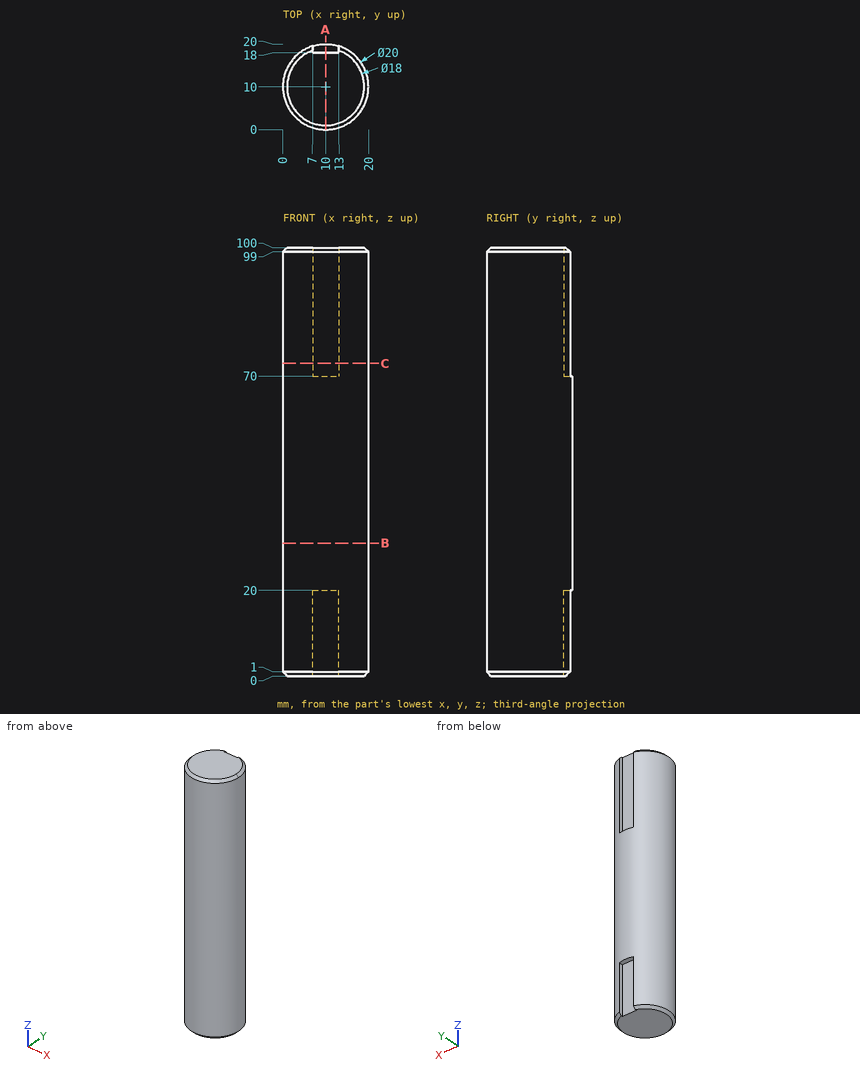
Job drawing, mm, ordinate dimensions from the low corner. One solid piece. Give positions to 0.01 mm unless a question says otherwise; leave off trailing zeros. Order: outer loops, then holes, each group sorted by start corner. A loop starts at its lowest first (then second) coordinate and runs counter-clockwise, first axis right, second up. Notation, with made-up numbers: (-14.5, -35.75) -> (-6.5, -35.75) arc R29 cw to (-6.5, 2.25) -> close; hole circle Ø7 at (45, 73). An arc over 180 degrees is marked (long way). Return JSON: item names as keys, results as strings.
Q1. Saw through at B-B (z = 31). Write the cut outline in (x, y).
Working result:
{"outline": "circle Ø20 at (10, 10)"}
Q2. Drill centre lines: line 1 (Y direction, x = 9.5, z = 54.5); line 2 (Y direction, x = 17.25, z = 61). Where is each one in solid material? Low to high.
Working result:
{"line 1": "0.01 to 19.99", "line 2": "3.11 to 16.89"}
Q3. Saw through at C-C (z = 73). Write the cut outline in (x, y), then the cut area to 3 significant figures.
Working result:
{"outline": "(7, 18) -> (7, 19.54) arc R10 ccw (long way) to (13, 19.54) -> (13, 18) -> close", "area": "303 mm²"}
Q4. Flat gauge pins, fed straight in: pin 1 (8 mm diameter, centred on x = 6, y = 17, fed in from -Z); pin 2 (0.5 mm diameter, centred on y = 19, z = 78.5, fed in from +X); pin 3 (0.5 mm diameter, centred on y = 18.5, z = 87, fed in from -X); pin 4 (1 mm diameter, centred on x = 2.5, z = 53, fed in from +Y). Where does each tip first touch, or does it go through?
Working result:
{"pin 1": "z = 0", "pin 2": "x = 14.84", "pin 3": "x = 4.35", "pin 4": "y = 17.14"}
Q5. Saw through at A-A (x = 10). Write the cut outline in (y, z), then the cut area to 3 significant figures.
Working result:
{"outline": "(0, 1) -> (1, 0) -> (18, 0) -> (18, 20) -> (20, 20) -> (20, 70) -> (18, 70) -> (18, 100) -> (1, 100) -> (0, 99) -> close", "area": "1,900 mm²"}
